```python
from build123d import *

# Parameters (mm, degrees)
F0_R     = 3.647768
F1_DEPTH = 660


with BuildPart() as f1:
    # F0 (on Front) → F1 (new body)
    with BuildSketch(Plane.XZ):
        with BuildLine():
            Line((-4.15, 22.5), (-22.5, 22.5))
            Line((-22.5, 22.5), (-22.5, 4.15))
            Line((-22.5, 4.15), (-18, 4.15))
            Line((-18, 4.15), (-18, 5.75))
            ThreePointArc((-18, 5.75), (-18.5, 6.25), (-18, 6.75))
            Line((-18, 6.75), (-9.8, 6.75))
            Line((-9.8, 6.75), (-7.2, 4.15))
            Line((-7.2, 4.15), (-7.2, -4.15))
            Line((-7.2, -4.15), (-9.8, -6.75))
            Line((-9.8, -6.75), (-18, -6.75))
            ThreePointArc((-18, -6.75), (-18.5, -6.25), (-18, -5.75))
            Line((-18, -5.75), (-18, -4.15))
            Line((-18, -4.15), (-22.5, -4.15))
            Line((-22.5, -4.15), (-22.5, -22.5))
            Line((-22.5, -22.5), (-4.15, -22.5))
            Line((-4.15, -22.5), (-4.15, -18))
            Line((-4.15, -18), (-5.75, -18))
            ThreePointArc((-5.75, -18), (-6.25, -18.5), (-6.75, -18))
            Line((-6.75, -18), (-6.75, -9.8))
            Line((-6.75, -9.8), (-4.15, -7.2))
            Line((-4.15, -7.2), (4.15, -7.2))
            Line((4.15, -7.2), (6.75, -9.8))
            Line((6.75, -9.8), (6.75, -18))
            ThreePointArc((6.75, -18), (6.25, -18.5), (5.75, -18))
            Line((5.75, -18), (4.15, -18))
            Line((4.15, -18), (4.15, -22.5))
            Line((4.15, -22.5), (22.5, -22.5))
            Line((22.5, -22.5), (22.5, -4.15))
            Line((22.5, -4.15), (18, -4.15))
            Line((18, -4.15), (18, -5.75))
            ThreePointArc((18, -5.75), (18.5, -6.25), (18, -6.75))
            Line((18, -6.75), (9.8, -6.75))
            Line((9.8, -6.75), (7.2, -4.15))
            Line((7.2, -4.15), (7.2, 4.15))
            Line((7.2, 4.15), (9.8, 6.75))
            Line((9.8, 6.75), (18, 6.75))
            ThreePointArc((18, 6.75), (18.5, 6.25), (18, 5.75))
            Line((18, 5.75), (18, 4.15))
            Line((18, 4.15), (22.5, 4.15))
            Line((22.5, 4.15), (22.5, 22.5))
            Line((22.5, 22.5), (4.15, 22.5))
            Line((4.15, 22.5), (4.15, 18))
            Line((4.15, 18), (5.75, 18))
            ThreePointArc((5.75, 18), (6.25, 18.5), (6.75, 18))
            Line((6.75, 18), (6.75, 9.8))
            Line((6.75, 9.8), (4.15, 7.2))
            Line((4.15, 7.2), (-4.15, 7.2))
            Line((-4.15, 7.2), (-6.75, 9.8))
            Line((-6.75, 9.8), (-6.75, 18))
            ThreePointArc((-6.75, 18), (-6.25, 18.5), (-5.75, 18))
            Line((-5.75, 18), (-4.15, 18))
            Line((-4.15, 18), (-4.15, 22.5))
        make_face()
        with BuildLine():
            Line((-8.9, -12.1), (-8.9, -19.5))
            ThreePointArc((-8.9, -19.5), (-9.192893, -20.207107), (-9.9, -20.5))
            Line((-9.9, -20.5), (-19.5, -20.5))
            ThreePointArc((-19.5, -20.5), (-20.207107, -20.207107), (-20.5, -19.5))
            Line((-20.5, -19.5), (-20.5, -9.9))
            ThreePointArc((-20.5, -9.9), (-20.207107, -9.192893), (-19.5, -8.9))
            Line((-19.5, -8.9), (-12.1, -8.9))
            Line((-12.1, -8.9), (-8.9, -12.1))
        make_face(mode=Mode.SUBTRACT)
        with BuildLine():
            Line((8.9, -12.1), (12.1, -8.9))
            Line((12.1, -8.9), (19.5, -8.9))
            ThreePointArc((19.5, -8.9), (20.207107, -9.192893), (20.5, -9.9))
            Line((20.5, -9.9), (20.5, -19.5))
            ThreePointArc((20.5, -19.5), (20.207107, -20.207107), (19.5, -20.5))
            Line((19.5, -20.5), (9.9, -20.5))
            ThreePointArc((9.9, -20.5), (9.192893, -20.207107), (8.9, -19.5))
            Line((8.9, -19.5), (8.9, -12.1))
        make_face(mode=Mode.SUBTRACT)
        with BuildLine():
            ThreePointArc((-20.5, 19.5), (-20.207107, 20.207107), (-19.5, 20.5))
            Line((-19.5, 20.5), (-9.9, 20.5))
            ThreePointArc((-9.9, 20.5), (-9.192893, 20.207107), (-8.9, 19.5))
            Line((-8.9, 19.5), (-8.9, 12.1))
            Line((-8.9, 12.1), (-12.1, 8.9))
            Line((-12.1, 8.9), (-19.5, 8.9))
            ThreePointArc((-19.5, 8.9), (-20.207107, 9.192893), (-20.5, 9.9))
            Line((-20.5, 9.9), (-20.5, 19.5))
        make_face(mode=Mode.SUBTRACT)
        Circle(F0_R, mode=Mode.SUBTRACT)
        with BuildLine():
            Line((12.1, 8.9), (8.9, 12.1))
            Line((8.9, 12.1), (8.9, 19.5))
            ThreePointArc((8.9, 19.5), (9.192893, 20.207107), (9.9, 20.5))
            Line((9.9, 20.5), (19.5, 20.5))
            ThreePointArc((19.5, 20.5), (20.207107, 20.207107), (20.5, 19.5))
            Line((20.5, 19.5), (20.5, 9.9))
            ThreePointArc((20.5, 9.9), (20.207107, 9.192893), (19.5, 8.9))
            Line((19.5, 8.9), (12.1, 8.9))
        make_face(mode=Mode.SUBTRACT)
    extrude(amount=F1_DEPTH)


solid = f1.part
```
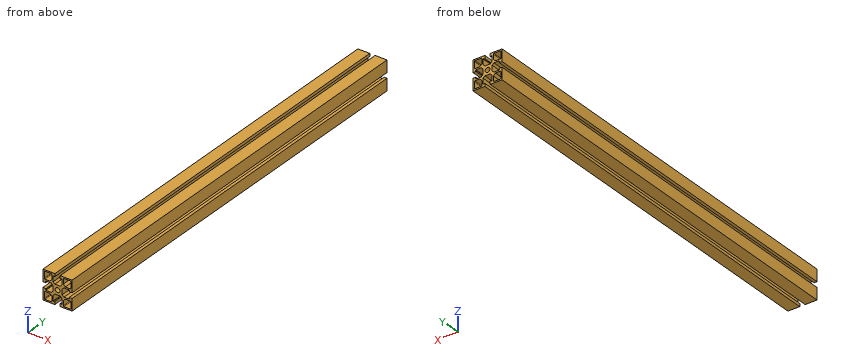
Input: part model. Units: mm. Frame: model coordinates. Give positions to 0.01 mm unless a question says otherwise; leave off trailing zeros. Write each question's results on one line, items separated by ' | '. Start each with the question number.
Item 1: Cut plane A-A on y = -454.5. Give the number of separate pieces and of enclosed holes in the cut face, then the cut area to 3 significant figures.
Item 2: Line query: line 1 (X direction, y = -430, z = -17.5); line 2 (Z direction, x = 0, y = -459). Output: solid intervals per line, ascending.
Item 3: Contact query for flat-ended pins moving along their axis: P1, Ø10, axis at x = 4.5, z = 14, coming from the -Y side; P2, Ø2.5, axis at x = 0, y = -403.5, coming from the +Z side. Output: stop coordinate, or through.
Established:
1) separate pieces: 1 | enclosed holes: 5 | area: 759 mm^2
2) line 1: -22.5 to -20.5, -8.9 to -6.75, 6.75 to 8.9, 20.5 to 22.5 | line 2: -7.2 to -3.65, 3.65 to 7.2
3) P1: y = -660 | P2: z = 7.2
